from build123d import *

# Parameters (mm, degrees)
F1_DEPTH = 76.2
F2_R     = 4.5085
F4_DEPTH = 76.2
F3_R     = 4.5085
F5_DEPTH = 76.2


with BuildPart() as f1:
    # F0 (on Front) → F1 (new body)
    with BuildSketch(Plane.XZ):
        Polygon((-31.118602, 76.344244), (-76.136798, 76.344244), (-76.136798, -25.309771), (-76.136798, -76.344237), (-76.136798, -76.551691), (42.113781, -76.551691), (42.113781, -25.309771), (-31.118602, -25.309771), align=None)
    extrude(amount=F1_DEPTH)

    # F2 (on face) → F4 (cut)
    with BuildSketch(Plane.XY.offset(-25.309771)):
        with Locations((-8.686219, -36.344424)):
            Circle(F2_R)
    extrude(amount=-F4_DEPTH, mode=Mode.SUBTRACT)

    # F3 (on face) → F5 (cut)
    with BuildSketch(Plane.YZ.offset(-31.118602)):
        with Locations((-42.6085, 8.335744)):
            Circle(F3_R)
    extrude(amount=-F5_DEPTH, mode=Mode.SUBTRACT)


solid = f1.part
Here's how the part is built. I have some questions about the finished solid (model axes, mm). A direction names the side the tool comes from. Give positions to 0.01 mm unless a question says otherwise; leave off trailing zeros. Order: outer loops, then holes, each group sorted by start corner. A loop starts at its lowest first (then second) coordinate and runs counter-clockwise, first axis right, second up. Notation, with made-up numbers: M 15.25,20.25 L 36.25,20.25 A26 ccw 36.25,59.25 Z; hole C -10.75,79 d6. An arc over 180 degrees is marked long. Answer as a JSON object with one key per item and string values. Group by question number.
1) Suppose I cut it at B-B, the plane z = 60. Write out the boundary of the cut face in (x, y).
2) We'd pull the mould along Y, two halves only. Please class faces 3 (the flat face through (-76.137, -38, 1)), 4 (the flat face through (-44, -76.2, -16)), 5 (the cylindrical face through (-12.01, -33.3, -50.57)): pulls with the +Y half, pulls with the -Y half, needs draft (parallel to the pull), parting line crosses it, or undercut.
3) Suppose I cut it at A-A, the plane y = -6.5. Write out the boundary of the cut face in (x, z).
4) Suppose I cut it at C-C, the plane x = 17.5. Write out the boundary of the cut face in (y, z).
5) Please list where these lines run through material, in increasing order: L1, parallel to X at y = -36, z = 37; L2, parallel to Z at x = 17, y = -62. Write a range as [from, to].
6) I'm going to push flat-ended pins straight in: pin 1 Ø22 at (x, y) = (21, -56) entering from +Z; pin 2 Ø23 at (y, z) = (-28, 2.5) entering from +X; pin 3 Ø5.5 at (y, z) = (-42.61, 8.34) entering from +X. Where does each tip first touch, or does it pass through?
7) On a 3-axis mill with a long thin cutter (end or side, diameter ignored), from which of +Z, -Z, +X, -X, +Y, -Y can I reach the whole of each face in a straight line? I mean faces 1 (the flat face through (-44, 0, -16)), 2 (the flat face through (6, -38, -25.31)). Say none if no direction works.
Results found:
{
 "1": {"outline": "M -76.14,-76.2 L -31.12,-76.2 L -31.12,0 L -76.14,0 Z"},
 "2": {"face 3": "needs draft", "face 4": "pulls with the -Y half", "face 5": "undercut"},
 "3": {"outline": "M -76.14,-76.55 L 42.11,-76.55 L 42.11,-25.31 L -31.12,-25.31 L -31.12,76.34 L -76.14,76.34 Z"},
 "4": {"outline": "M -76.2,-76.55 L 0,-76.55 L 0,-25.31 L -76.2,-25.31 Z"},
 "5": {"L1": "[-76.14, -31.12]", "L2": "[-76.55, -25.31]"},
 "6": {"pin 1": "z = -25.31", "pin 2": "x = -31.12", "pin 3": "through"},
 "7": {"face 1": "+Z, -Z, +X, -X, +Y", "face 2": "+Z, +X, +Y, -Y"}
}
